For this review, take the finished solid that the model builds, in its own axes (mm). A direction names the side the tool comes from. Coordinates: 2 decimals unless noted, no trailing zeros. Loops run counter-clockwise (first coordinate to the right, second up) from the corner with the lowest first, then second, coordinate; pieces in that order, holes last. Notation, with made-up numbers: M 43.5,42 L 63.5,42 A18 cw 63.5,59 Z; hole C -36.5,-38 d7. An arc over 180 degrees is marked long. Put each result on its own line as item: value.
```python
from build123d import *

# Parameters (mm, degrees)
SKETCH_4_W          = 9
SKETCH_4_H          = 10
EXTRUDE_2_DEPTH     = 10
CUT_EXTRUDE_1_DEPTH = 10
SKETCH_4_2_W        = 9
SKETCH_4_2_H        = 10
CUT_EXTRUDE_START   = 10
CUT_EXTRUDE_2_DEPTH = 10
SKETCH_8_R          = 1.5
CUT_EXTRUDE_3_DEPTH = 10
SKETCH_9_W          = 7.29
SKETCH_9_H          = 6
CUT_EXTRUDE_5_DEPTH = 110
SKETCH_13_W         = 7.29
SKETCH_13_H         = 6
CUT_EXTRUDE_6_DEPTH = 40


with BuildPart() as part:
    # 草图4 → 凸台-拉伸2 (new body)
    with BuildSketch(Plane(origin=(0, 0, 0), x_dir=(1, 0, 0), z_dir=(0, 1, 0))):
        with Locations((-19.8, -3.957142857)):
            Rectangle(SKETCH_4_W, SKETCH_4_H)
    extrude(amount=EXTRUDE_2_DEPTH)

    # 草图6 → 切除-拉伸1 (cut)
    with BuildSketch(Plane.XY.offset(8.957142857)):
        with BuildLine():
            Line((-24.3, 10), (-24.3, 5))
            ThreePointArc((-24.3, 5), (-19.8, 9.5), (-15.3, 5))
            Line((-15.3, 5), (-15.3, 10))
            Line((-15.3, 10), (-24.3, 10))
        make_face()
    extrude(amount=-CUT_EXTRUDE_1_DEPTH, mode=Mode.SUBTRACT)

    # 扫描2: sweep along a path in 草图5
    with BuildLine(Plane.XY.offset(3.957142857)) as sweep_2_path:
        Line((-19.8, 0), (-19.8, -110))
        Line((-19.8, -110), (5.372988935, -140))
    # 草图4<2> → 扫描2 (sweep)
    with BuildSketch(Plane(origin=(0, 0, 0), x_dir=(1, 0, 0), z_dir=(0, 1, 0))):
        with Locations((-19.8, -3.957142857)):
            Rectangle(SKETCH_4_2_W, SKETCH_4_2_H)
    sweep(path=sweep_2_path.line, transition=Transition.RIGHT)

    # 草图7 → 切除-拉伸2 (cut)
    with BuildSketch(Plane.XY.offset(3.957142857).offset(CUT_EXTRUDE_START)):
        with BuildLine():
            Line((-24.3, 5), (-24.3, 0.5))
            Line((-24.3, 0.5), (-15.3, 0.5))
            Line((-15.3, 0.5), (-15.3, 5))
            ThreePointArc((-15.3, 5), (-19.8, 9.5), (-24.3, 5))
        make_face()
    extrude(amount=-CUT_EXTRUDE_2_DEPTH, mode=Mode.SUBTRACT)

    # 草图8 → 切除-拉伸3 (cut)
    with BuildSketch(Plane.XY.offset(3.957142857)):
        with Locations((-19.8, 5)):
            Circle(SKETCH_8_R)
    extrude(amount=-CUT_EXTRUDE_3_DEPTH, mode=Mode.SUBTRACT)

    # 草图9 → 切除-拉伸5 (cut)
    with BuildSketch(Plane(origin=(0, -0.5, 0), x_dir=(1, 0, 0), z_dir=(0, 1, 0))):
        with Locations((-18.945, -3.957142857)):
            Rectangle(SKETCH_9_W, SKETCH_9_H)
    extrude(amount=-CUT_EXTRUDE_5_DEPTH, mode=Mode.SUBTRACT)

    # 草图13 → 切除-拉伸6 (cut)
    with BuildSketch(Plane(origin=(71.15653231, -84.801053017, 0), x_dir=(0.7660444431189772, 0.6427876096865404, 0), z_dir=(0.6427876096865403, -0.7660444431189771, 0))):
        with Locations((-85.019317039, 3.957142857)):
            Rectangle(SKETCH_13_W, SKETCH_13_H)
    extrude(amount=-CUT_EXTRUDE_6_DEPTH, mode=Mode.SUBTRACT)


solid = part.part
```
(1) Draft analysis for pull direction Y (two halves, no side actions). For faces 4 (the flat face through (-3.1, -122.9, 0)), 5 (the flat face through (-11.004, -127.484, 3.887)), 6 (the flat face through (-15.3, -52.5, 0.7)), 7 (the flat face through (-22.59, -55, 4)), state which applies: +Y half, -Y half, draft (parallel to the pull), parting line (faces both ways), or undercut.
Determined:
face 4: +Y half
face 5: -Y half
face 6: draft
face 7: undercut
(2) Add section B-B (y = -34). Write out the cut boundary in (x, z), plus the area to 3 significant figures.
Determined:
outline: M -24.3,-1.04 L -15.3,-1.04 L -15.3,0.96 L -22.59,0.96 L -22.59,6.96 L -15.3,6.96 L -15.3,8.96 L -24.3,8.96 Z
area: 46.3 mm^2
(3) Add section A-A (x = -19.8). Write out the cut boundary in (y, z), plus the area to 3 significant figures.
Determined:
outline: M -117,-1.04 L 3.5,-1.04 L 3.5,3.96 L 0.5,3.96 L 0.5,8.96 L -117,8.96 Z; M 6.5,-1.04 L 9.5,-1.04 L 9.5,3.96 L 6.5,3.96 Z; hole M -114.34,0.96 L -0.5,0.96 L -0.5,6.96 L -114.34,6.96 Z
area: 522 mm^2
(4) Wall thickness on line 1 along Z through (x, y) = (-16, -29); line 2 along Y through (x, z) = (-19.8, 1.45); line 3 along Y through (x, z) = (-18, 1.75): over which ranges is each line inside the solid? List them lowest first. Write a range as [from, to].
Determined:
line 1: z = [-1.04, 0.96], [6.96, 8.96]
line 2: y = [-117, -114.34], [-0.5, 3.5], [6.5, 9.5]
line 3: y = [-119.15, -116.49], [-0.5, 9.12]
(5) Tool access review of faces 1 (the cylindrical face through (-19.9, 9.5, 1.5)), 2 (the flat face through (-20, 3, 3.957)), 3 (the flat face through (-19, -0.5, 4)): name each direction out of +Z, -Z, +X, -X, +Y, -Y from which nothing blocks a thin tool from reaching the whole face with its end or side.
Determined:
face 1: +Z, -Z, +Y
face 2: +Z, +X, -X, +Y
face 3: +X
(6) Add section C-C (x = -3.5). Write out the cut boundary in (y, z).
Determined:
outline: M -136.43,-1.04 L -122.42,-1.04 L -122.42,0.96 L -133.77,0.96 L -133.77,6.96 L -122.42,6.96 L -122.42,8.96 L -136.43,8.96 Z
(7) For pin 1 (7 mm diameter, centred on x = -18.5, y = 5, fed in from +Z); pin 2 (1 mm diameter, centred on y = -26, z = 6.5, fed in from +X); pin 3 (3 mm diameter, centred on y = -40.5, z = 5, fed in from +X), all flat-tipped, find the tip position at first contact; note any pin that passes through.
Determined:
pin 1: stops at z = 3.96
pin 2: stops at x = -15.3
pin 3: stops at x = -22.59
